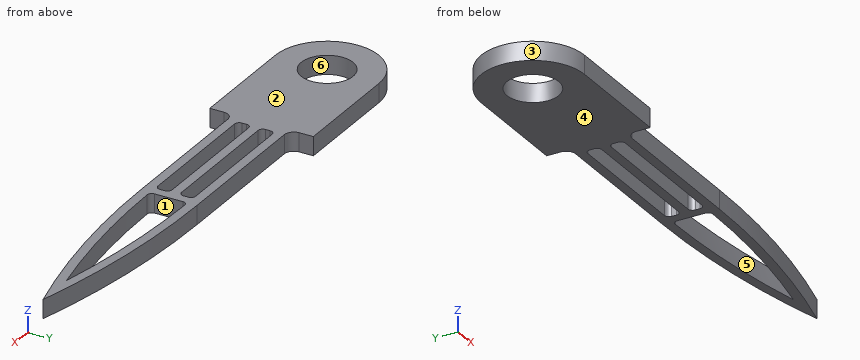
```python
from build123d import *

# Parameters (mm, degrees)
BOSS_EXTRUDE1_DEPTH = 5.08
SKETCH2_R           = 6.985
CUT_EXTRUDE1_DEPTH  = 133.913858194
FILLET1_R           = 2.54
SKETCH3_W           = 38.1
SKETCH3_H           = 3.81
CUT_EXTRUDE2_DEPTH  = 133.913858194
FILLET2_R           = 1.27


with BuildPart() as part:
    # Sketch1 → Boss-Extrude1 (new body)
    with BuildSketch(Plane.XY):
        with BuildLine():
            Line((0, 13.97), (30.48, 13.97))
            Line((30.48, 13.97), (30.48, 7.62))
            Line((30.48, 7.62), (73.66, 7.62))
            ThreePointArc((73.66, 7.62), (103.117430302, 5.706965649), (132.08, 0))
            ThreePointArc((132.08, 0), (103.117430302, -5.706965649), (73.66, -7.62))
            Line((73.66, -7.62), (30.48, -7.62))
            Line((30.48, -7.62), (30.48, -13.97))
            Line((30.48, -13.97), (0, -13.97))
            ThreePointArc((0, -13.97), (-13.97, 0), (0, 13.97))
        make_face()
    extrude(amount=BOSS_EXTRUDE1_DEPTH)

    # Sketch2 → Cut-Extrude1 (cut, through all)
    with BuildSketch(Plane.XY.offset(5.08)):
        Circle(SKETCH2_R)
    extrude(amount=-CUT_EXTRUDE1_DEPTH, mode=Mode.SUBTRACT)

    # Fillet1
    fillet1_edges = [part.edges().sort_by_distance(p)[0] for p in [
        (30.48, -7.62, 2.54),
        (30.48, 7.62, 2.54),
    ]]
    fillet(fillet1_edges, radius=FILLET1_R)

    # Sketch3 → Cut-Extrude2 (cut, through all)
    with BuildSketch(Plane.XY.offset(5.08)):
        with Locations((52.07, -3.175)):
            Rectangle(SKETCH3_W, SKETCH3_H)
        with Locations((52.07, 3.175)):
            Rectangle(SKETCH3_W, SKETCH3_H)
        with BuildLine():
            Line((73.66, -5.08), (73.66, 5.08))
            ThreePointArc((73.66, 5.08), (97.577396737, 3.806398837), (121.224283519, 0))
            ThreePointArc((121.224283519, 0), (97.577396737, -3.806398837), (73.66, -5.08))
        make_face()
    extrude(amount=-CUT_EXTRUDE2_DEPTH, mode=Mode.SUBTRACT)

    # Fillet2
    fillet2_edges = [part.edges().sort_by_distance(p)[0] for p in [
        (73.66, -5.08, 2.54),
        (73.66, 5.08, 2.54),
        (71.12, 1.27, 2.54),
        (33.02, 1.27, 2.54),
        (33.02, 5.08, 2.54),
        (71.12, 5.08, 2.54),
        (71.12, -1.27, 2.54),
        (71.12, -5.08, 2.54),
        (33.02, -5.08, 2.54),
        (33.02, -1.27, 2.54),
    ]]
    fillet(fillet2_edges, radius=FILLET2_R)


solid = part.part
```
Verification items for the finished model (mm, model axes). Face numbers are marked on the shaded views. A direction names the side the tool comes from. Give positions to 0.01 mm unless a question says otherwise; leave off trailing zeros. Order: outer loops, then holes, each group sorted by start corner. A loop starts at its lowest first (then second) coordinate and runs counter-clockwise, first axis right, second up. Notation, with made-up numbers: (20, 37.25) -> (62, 37.25) arc R12 cw to (62, 44.25) -> close; hole circle Ø8 at (6.5, 29.5). An arc over 180 degrees is marked (long way). Use a Markdown table: item, result.
1) Material ranges on probe 1 along Y at (x, z) = (46, 2.75); probe 2 along Y at (x, z) = (0, 3.6) (3 decimals); probe 3 along Y at (x, z) = (1, 0.7), recorded low to high.
Results:
| item | result |
|---|---|
| probe 1 | -7.62 to -5.08, -1.27 to 1.27, 5.08 to 7.62 |
| probe 2 | -13.97 to -6.985, 6.985 to 13.97 |
| probe 3 | -13.97 to -6.91, 6.91 to 13.97 |
2) Section check A-A, the plane z = 0.9. Give the number of separate pieces and of enclosed holes in the cut face, then the cut area to 3 significant figures.
Results:
| item | result |
|---|---|
| separate pieces | 1 |
| enclosed holes | 4 |
| area | 1,650 mm² |
3) Section check C-C, the plane x = -3. Record the boundary of the cut face in (y, z), then the cut area to 3 significant figures.
Results:
| item | result |
|---|---|
| outline | (-13.64, 0) -> (-6.31, 0) -> (-6.31, 5.08) -> (-13.64, 5.08) -> close; (6.31, 0) -> (13.64, 0) -> (13.64, 5.08) -> (6.31, 5.08) -> close |
| area | 74.5 mm² |
4) Section check B-B, the plane x = 107.5. Record the boundary of the cut face in (y, z).
Results:
| item | result |
|---|---|
| outline | (-5.09, 0) -> (-2.52, 0) -> (-2.52, 5.08) -> (-5.09, 5.08) -> close; (2.52, 0) -> (5.09, 0) -> (5.09, 5.08) -> (2.52, 5.08) -> close |
5) Depth check by flat-ended pin: pin 1 Ø2.5 at (x, z) = (50.5, 2) entering from +Y; pin 2 Ø8 at (x, y) = (91, -3) entering from -Z; pin 3 Ø0.6 at (y, z) = (-3.5, 3.5) entering from -X; pin 4 Ø1.5 at (x, z) = (63, 3.5) entering from -Y. Enter the tip coordinate at first touch or a pass-through.
Results:
| item | result |
|---|---|
| pin 1 | y = 7.62 |
| pin 2 | z = 0 |
| pin 3 | x = -13.6 |
| pin 4 | y = -7.62 |
6) Tool access check on the marked faces 1 and 2. Record the directions out of +Z, -Z, +X, -X, +Y, -Y that give a thin tool (end or side, any length) a straight path to the whole face; none if there is none.
Results:
| item | result |
|---|---|
| face 1 | +Z, -Z |
| face 2 | +Z, +X, -X, +Y, -Y |
7) Mould release check, pull along Y, two halves, no side actions. Record for the marked faces 3, 4, 5 and 6: pulls with the +Y half, pulls with the -Y half, needs draft (parallel to the pull), parting line crosses it, or undercut.
Results:
| item | result |
|---|---|
| face 3 | parting line crosses it |
| face 4 | needs draft |
| face 5 | undercut |
| face 6 | undercut |
